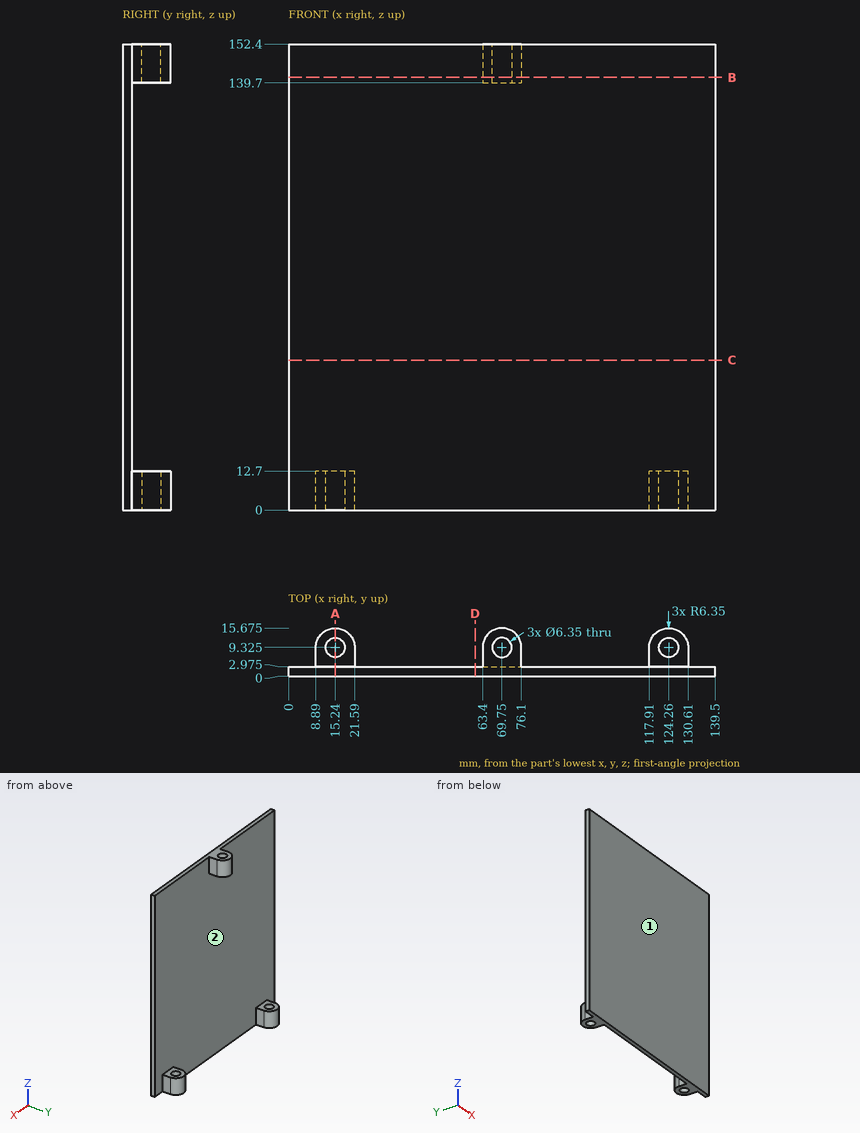
The figure shows three views and two pictorial views of one solid part (mm, origin at its lowest corner). Answer the questions. Give positions to 0.01 mm unless a question says otherwise; leave off trailing zeros. Loops run counter-clockwise (first coordinate to the right, second up) from the corner with the lowest first, then second, coordinate; pieces in that order, holes last. Notation, with made-up numbers: M -22.5,-8 L -17.5,-8 A21 ccw -17.5,26 Z; hole C 61,23 d11. An arc over 180 degrees is marked long. Write each question's results on one line, items separated by ' | '.
1. Given pin 1 (1 mm diameter, centred on x = 55, z = 60, fed in from +Y) (3 decimals); pin 2 (5 mm diameter, centred on y = 6, z = 7, fed in from +X); pin 3 (5 mm diameter, centred on x = 15.24, y = 9.325, fed in from -Z) (3 decimals); pin 4 (6.5 mm diameter, centred on x = 68.5, y = 7.5, fed in from -Z), each flat-ended and moving along its own axis, determine where each tip first touches the part or whether it passes through.
Values:
pin 1: stops at y = 2.975 | pin 2: stops at x = 130.61 | pin 3: passes through | pin 4: stops at z = 139.7
2. Section B-B on z = 141.5 is taken. Give the vertices of the cut face in (x, y) (3 decimals), plus the area to 3 significant figures.
Values:
outline: M 0,0 L 139.5,0 L 139.5,2.975 L 76.1,2.975 L 76.1,9.325 A6.35 ccw 63.4,9.325 L 63.4,2.975 L 0,2.975 Z; hole C 69.75,9.325 d6.35 | area: 527 mm^2
3. Straight lines are drawn through the part: line 1 (Y direction, x = 69.75, z = 146) (3 decimals); line 2 (Y direction, x = 53, z = 53) (3 decimals); line 3 (Z direction, x = 76, y = 5.5). For each, find the intervals that lie inside material, in ascending order. Write a range as [from, to].
Values:
line 1: y = [0, 6.15], [12.5, 15.675] | line 2: y = [0, 2.975] | line 3: z = [139.7, 152.4]
4. Section D-D on x = 61 is taken. Give the vertices of the cut face in (y, z) (3 decimals), plus the area to 3 significant figures.
Values:
outline: M 0,0 L 2.975,0 L 2.975,152.4 L 0,152.4 Z | area: 453 mm^2
5. The mould has two halves that part along Y. Classify the marked faces 1 and 2: pulls with the +Y half, pulls with the -Y half, needs draft (parallel to the pull), parting line crosses it, or undercut.
Values:
face 1: pulls with the -Y half | face 2: pulls with the +Y half
6. Section C-C on z = 49 is taken. Give the vertices of the cut face in (x, y) (3 decimals), plus the area to 3 significant figures.
Values:
outline: M 0,0 L 139.5,0 L 139.5,2.975 L 0,2.975 Z | area: 415 mm^2
7. Section A-A on x = 15.24 is taken. Give the vertices of the cut face in (y, z) (3 decimals), plus the area to 3 significant figures.
Values:
outline: M 0,0 L 6.15,0 L 6.15,12.7 L 2.975,12.7 L 2.975,152.4 L 0,152.4 Z; M 12.5,0 L 15.675,0 L 15.675,12.7 L 12.5,12.7 Z | area: 534 mm^2
